Autodesk Inventor part; units mm, degrees
ref_plane "YZ Plane" through (0, 0, 0) normal (1, 0, 0) x (0, 1, 0)
ref_plane "XZ Plane" through (0, 0, 0) normal (0, 1, 0) x (-1, 0, 0)
ref_plane "XY Plane" through (0, 0, 0) normal (0, 0, 1) x (1, 0, 0)
sketch "Sketch1" plane through (0, 0, 0) normal (0, 0, 1) x (1, 0, 0)
  circle A0 centre (0, 0) radius 12.35
  circle A1 centre (7.4246, 7.4246) radius 12.2
  line L0 (-13.413, -13.413) -> (25.4094, 25.4094) construction
  line L1 (-10.6165, 0) -> (15.2552, 0) construction
  line L2 (7.4246, 7.4246) -> (15.8638, 6.41) construction
  line L3 (16.6649, 18.5138) -> (22.6753, 24.5242) construction
  circle A2 centre (15.8638, 6.41) radius 1.5
  line L4 (7.4246, 7.4246) -> (-1.0146, 8.4392) construction
  circle A3 centre (-1.0146, 8.4392) radius 1.5
  line L5 (0, 0) -> (-1.0146, 8.4392) construction
  line L6 (0, 0) -> (1.0146, -8.4392) construction
  circle A4 centre (1.0146, -8.4392) radius 1.5
  circle A5 centre (-9.8288, -9.8288) radius 12.2
  line L7 (-5.2409, -11.1828) -> (0, 0)
  point P0 (11.6813, -4.0087)
  point P1 (-0.7603, -1.6223)
  dimension "d0" = 24.7
  dimension "d1" = 24.4
  dimension "d2" = 0
  dimension "d3" = 45
  dimension "d4" = 0
  dimension "d5" = 10.5
  dimension "d20" = 8.5
  dimension "d21" = 3
  dimension "d22" = 3
  dimension "d23" = 3
  dimension "d24" = 24.4
  dimension "d25" = 24.4
  dimension "d26" = 4.5
extrude "Extrusion1" add sketch "Sketch1" along normal blind 3 contours A0 A5 A4 L7 A1 | A0 L7 A5 A4
sketch "Sketch3" plane through (0, 0, 3) normal (0, 0, 1) x (1, 0, 0)
  circle A0 centre (0, 0) radius 12.35
  circle A1 centre (7.4246, 7.4246) radius 12.2
  line L0 (-13.413, -13.413) -> (25.4094, 25.4094) construction
  line L1 (-10.6165, 0) -> (15.2552, 0) construction
  line L2 (7.4246, 7.4246) -> (15.8638, 6.41) construction
  line L3 (16.6649, 18.5138) -> (22.6753, 24.5242) construction
  circle A2 centre (15.8638, 6.41) radius 1.5
  line L4 (7.4246, 7.4246) -> (-1.0146, 8.4392) construction
  circle A3 centre (-1.0146, 8.4392) radius 1.5
  line L5 (0, 0) -> (-1.0146, 8.4392) construction
  line L6 (0, 0) -> (1.0146, -8.4392) construction
  circle A4 centre (1.0146, -8.4392) radius 1.5
  circle A5 centre (-9.8288, -9.8288) radius 12.2
  line L7 (-5.2409, -11.1828) -> (0, 0)
  point P0 (11.6813, -4.0087)
  point P1 (-0.7603, -1.6223)
  point P2 (-0.7743, -1.6522)
  point P3 (2.1356, -7.4425)
  point P4 (2.3507, -9.1211)
  point P5 (2.146, -12.1621)
  dimension "d32" = 24.7
  dimension "d33" = 24.4
  dimension "d34" = 0
  dimension "d35" = 45
  dimension "d36" = 0
  dimension "d37" = 10.5
  dimension "d38" = 8.5
  dimension "d39" = 3
  dimension "d40" = 3
  dimension "d41" = 3
  dimension "d42" = 24.4
  dimension "d43" = 24.4
  dimension "d44" = 4.5
extrude "Extrusion3" add sketch "Sketch3" along normal blind 15.5 contours A0 A5 A4 L7 A1 | A4 A5 picked at (2.3363, -8.2121)
sketch "Sketch4" plane through (0, 0, 3) normal (0, 0, 1) x (1, 0, 0)
  line L0 (-2.1493, -8.7099) -> (-0.8017, -5.8346)
  line L1 (-0.8017, -5.8346) -> (2.3621, -5.5639)
  line L2 (2.3621, -5.5639) -> (4.1785, -8.1686)
  line L3 (4.1785, -8.1686) -> (2.8309, -11.0439)
  line L4 (2.8309, -11.0439) -> (-0.3329, -11.3146)
  line L5 (-0.3329, -11.3146) -> (-2.1493, -8.7099)
  point P0 (0, 0)
  point P1 (1.0146, -8.4392)
  dimension "d49" = 5.5
extrude "Extrusion4" cut sketch "Sketch4" along normal blind 2 and the other way blind 1
sketch "Sketch5" plane through (0, 0, 18.5) normal (0, 0, 1) x (1, 0, 0)
  circle A0 centre (0, 0) radius 12.35
  circle A1 centre (7.4246, 7.4246) radius 12.2
  line L0 (-13.413, -13.413) -> (25.4094, 25.4094) construction
  line L1 (-10.6165, 0) -> (15.2552, 0) construction
  line L2 (7.4246, 7.4246) -> (15.8638, 6.41) construction
  line L3 (16.6649, 18.5138) -> (22.6753, 24.5242) construction
  circle A2 centre (15.8638, 6.41) radius 1.5
  line L4 (7.4246, 7.4246) -> (-1.0146, 8.4392) construction
  circle A3 centre (-1.0146, 8.4392) radius 1.5
  line L5 (0, 0) -> (-1.0146, 8.4392) construction
  line L6 (0, 0) -> (1.0146, -8.4392) construction
  circle A4 centre (1.0146, -8.4392) radius 1.5
  circle A5 centre (-9.8288, -9.8288) radius 12.2
  line L7 (-5.2409, -11.1828) -> (0, 0)
  line L8 (-31.042, -9.8288) -> (7.4246, 28.6378)
  line L9 (7.4246, 28.6378) -> (28.6378, 7.4246)
  line L10 (28.6378, 7.4246) -> (-9.8288, -31.042)
  line L11 (-9.8288, -31.042) -> (-31.042, -9.8288)
  circle A6 centre (-9.8288, -9.8288) radius 15
  circle A7 centre (7.4246, 7.4246) radius 15
  point P0 (11.6813, -4.0087)
  point P1 (-0.7603, -1.6223)
  point P2 (2.146, -12.1621)
  point P3 (-12.1621, 2.146)
  point P4 (-4.0087, 11.6813)
  point P5 (0.7778, -20.4354)
  point P6 (18.0312, -3.182)
  point P7 (-3.182, 18.0312)
  point P8 (-20.4354, 0.7778)
  dimension "d54" = 24.7
  dimension "d55" = 24.4
  dimension "d56" = 0
  dimension "d57" = 45
  dimension "d58" = 0
  dimension "d59" = 10.5
  dimension "d60" = 8.5
  dimension "d61" = 3
  dimension "d62" = 3
  dimension "d63" = 3
  dimension "d64" = 24.4
  dimension "d65" = 24.4
  dimension "d66" = 4.5
  dimension "d67" = 15
  dimension "d68" = 15
  dimension "d69" = 30
  dimension "d70" = 15
extrude "Extrusion5" add sketch "Sketch5" against normal blind 18.5 contours A0 A7 A1 | A0 A6 L8 A7 | A7 L10 A6 A0 | A0 A5 A6
fillet "Fillet1" radius 3 1 edges at (-5.2409, -11.1828, 1.5)
fillet "Fillet2" radius 3 1 edges at (-0.7603, -1.6223, 9.25)
properties part number "Hiolder_28"
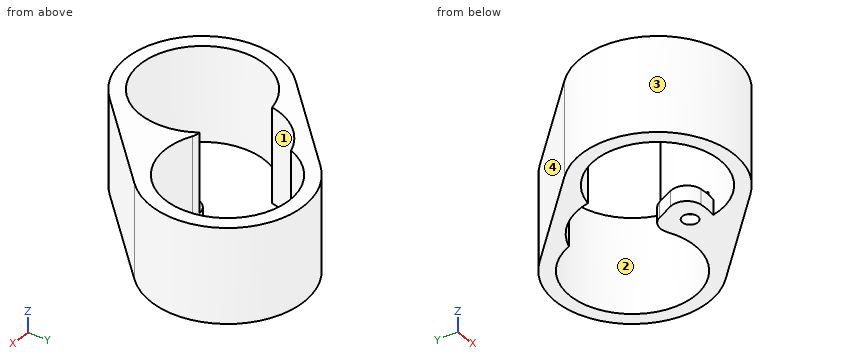
For this review, take the finished solid that the model builds, in its own axes (mm). Face numbers are marked on the shaded views. Round coordinates to 2 decimals unless told otherwise and drop trailing zeros. Order: outer loops, then holes, each group sorted by start corner. A loop starts at its lowest first (then second) coordinate and runs counter-clockwise, first axis right, second up. Notation, with made-up numbers: (-18, -24) -> (-1, -24) arc R24 cw to (-1, 4) -> close; hole circle Ø6 at (83.5, 16). An arc over 180 degrees is marked (long way). Put each result on its own line as item: value.
Q1. Add section A-A on y = -15.5. Write out the cut boundary in (x, z).
Check result:
outline: (-23.72, 0) -> (-20.63, 0) -> (-20.63, 18.5) -> (-23.72, 18.5) -> close; (0.97, 0) -> (5.71, 0) -> (5.71, 18.5) -> (0.97, 18.5) -> close
Q2. Insertion check: pin 1 Ø12 at (x, y) = (-11, -11.5) entering from +Z; pin 2 Ø2 at (x, z) = (2, 11) entering from -Y; pin 3 Ø8 at (x, z) = (17, 7.5) entering from -Y; pin 4 Ø4 at (y, z) = (15.5, 6.5) entering from +X. Each pin has a flat end and moves straight along its axis. Give the tip position at first contact, or say it passes through.
Check result:
pin 1: through
pin 2: y = -20.21
pin 3: y = -8.21
pin 4: x = 21.14
Q3. For probe 1 along Y at (x, z) = (7, 7.25); probe 2 along X at (y, z) = (10.5, 3.5); probe 3 along X at (y, z) = (2.5, 16.75), list the stretches that pass through material, from the lowest coordinate up. Write a range as [from, to].
Check result:
probe 1: [-14.21, -4.77], [19.62, 22.42]
probe 2: [-10.71, -6.5], [19.23, 22.11]
probe 3: [-18.71, -12.09], [18.59, 21.59]
Q4. Mouldability with a two-part tool opening along Y and no side actions: class the marked faces 1, 2, 3 and 4 as pulls with the +Y half, pulls with the -Y half, needs draft (parallel to the pull), parting line crosses it, or undercut.
Check result:
face 1: undercut
face 2: undercut
face 3: parting line crosses it
face 4: pulls with the +Y half
Q5. Add section B-B on x = 17. Write out the cut boundary in (y, z), plus the area to 3 significant figures.
Check result:
outline: (-4.21, 0) -> (-0.14, 0) -> (-0.14, 18.5) -> (-4.21, 18.5) -> close; (14.98, 0) -> (18.97, 0) -> (18.97, 18.5) -> (14.98, 18.5) -> close
area: 149 mm2
